Read the model definition and answer for the solid it produces. Units are mm, in the model's axes. Face numbers are marked on the shaded views. A direction names the side the tool comes from. Round coordinates to 2 decimals unless told otherwise and drop trailing zeros. Loops run counter-clockwise (first coordinate to the right, second up) from the corner with the lowest first, then second, coordinate; pieces in that order, holes last. Notation, with made-up numbers: M 6.5,76.5 L 25.5,76.5 A23 ccw 25.5,96.5 Z; hole C -9,-28.75 d1. An arc over 180 degrees is marked long. Write each question's results on one line, items separated by ' | '.
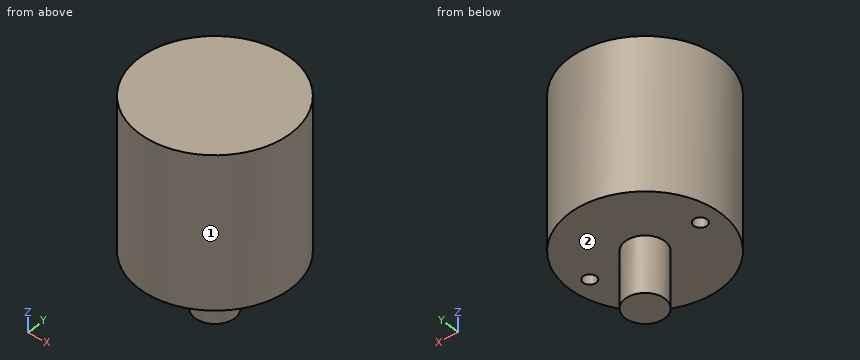
Autodesk Inventor part; units mm, degrees
ref_plane "YZ Plane" through (0, 0, 0) normal (1, 0, 0) x (0, 1, 0)
ref_plane "XZ Plane" through (0, 0, 0) normal (0, 1, 0) x (-1, 0, 0)
ref_plane "XY Plane" through (0, 0, 0) normal (0, 0, 1) x (1, 0, 0)
sketch "Sketch1" plane through (0, 0, 0) normal (0, 0, 1) x (1, 0, 0)
  circle A0 centre (0, 0) radius 11.5
  dimension "d0" = 23
extrude "Extrusion1" add sketch "Sketch1" along normal blind 23
sketch "Sketch2" plane through (0, 0, 0) normal (0, 0, -1) x (-1, 0, 0)
  circle A0 centre (8.5, 0) radius 1
  circle A1 centre (-8.5, 0) radius 1
  point P0 (0, 0)
  dimension "d3" = 2
  dimension "d4" = 8.5
  dimension "d7" = 360
extrude "Extrusion2" cut sketch "Sketch2" against normal blind 8
sketch "Sketch3" plane through (0, 0, 0) normal (0, 0, -1) x (-1, 0, 0)
  circle A0 centre (0, 0) radius 3
  dimension "d11" = 6
extrude "Extrusion3" add sketch "Sketch3" along normal blind 8.5
properties part number "AEAT-6012"
1. Find section D-D, the plane z = -6. Give the vertices of the cut face in (x, y).
Completed:
outline: C 0,0 d6
2. Which of the six approach directions +Z, -Z, +X, -X, +Y, -Y give full straight-line access (tool end or side, diameter ignored) to the marked faces 1 and 2?
Completed:
face 1: +Z, -Z | face 2: -Z
3. Find section A-A, the plane x = 0. Give the vertices of the cut face in (y, z).
Completed:
outline: M -11.5,0 L -3,0 L -3,-8.5 L 3,-8.5 L 3,0 L 11.5,0 L 11.5,23 L -11.5,23 Z
4. Find section B-B, the plane y = 0. Give the vertices of the cut face in (x, z).
Completed:
outline: M -11.5,0 L -9.5,0 L -9.5,8 L -7.5,8 L -7.5,0 L -3,0 L -3,-8.5 L 3,-8.5 L 3,0 L 7.5,0 L 7.5,8 L 9.5,8 L 9.5,0 L 11.5,0 L 11.5,23 L -11.5,23 Z
5. Given P1, Ø3, axis at x = 8.5, z = 7, coming from the +Y side; P2, Ø2, axis at y = -5.5, z = 0.5, coming from the -X side; P3, Ø1.5, axis at y = 4.5, z = 19.5, coming from the -X side, each flat-ended and moving along its own axis, determine where each tip first touches the part or whether it passes through.
Completed:
P1: stops at y = 9.12 | P2: stops at x = -10.58 | P3: stops at x = -10.87
6. Find the intervals of material crossed by L1, parallel to Z at x = -8.5, y = 0.25; L2, parallel to Z at x = -4.5, y = -1; L3, parallel to Y at x = 8.5, z = 2.75, in increasing order.
Completed:
L1: z = 8 to 23 | L2: z = 0 to 23 | L3: y = -7.75 to -1, 1 to 7.75
7. Find section C-C, the plane z = 5. Give the vertices of the cut face in (x, y), then the cut area to 3 significant figures.
Completed:
outline: C 0,0 d23; hole C -8.5,0 d2; hole C 8.5,0 d2 | area: 409 mm2
